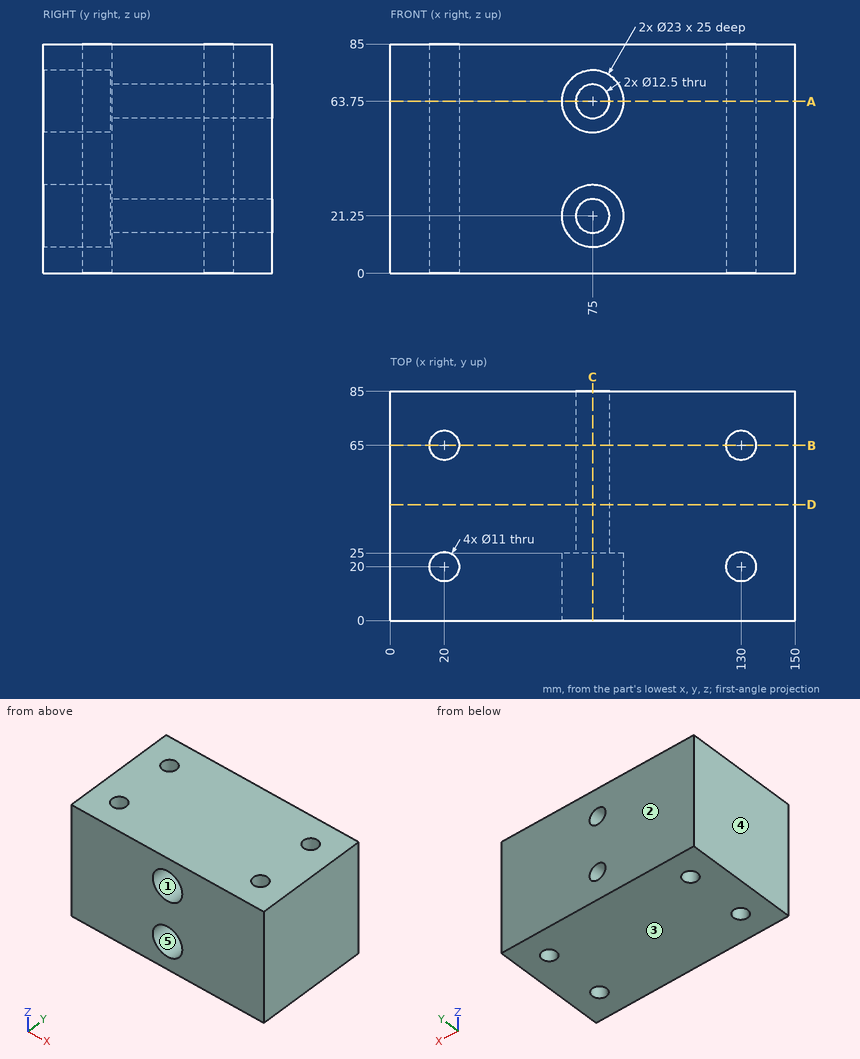
The figure shows three views and two pictorial views of one solid part (mm, origin at its lowest corner). Answer the questions. A direction names the side the tool comes from. Give positions to 0.01 mm unless a question says otherwise; leave off trailing zeros. Loops run counter-clockwise (first coordinate to the right, second up) from the corner with the lowest first, then second, coordinate; pieces in that order, holes last. Notation, with made-up numbers: (67.5, 88.25) -> (110.5, 88.25) arc R21 ccw to (110.5, 97.25) -> close; hole circle Ø9 at (-11.5, -13). An arc over 180 degrees is marked (long way). Use a Markdown table: item, result. Add a question column.
1. Flat-ended cylindrical pins translate along their axes: pin 1 Ø14.5 at (x, y) = (130, 65) entering from +Z; pin 2 Ø7 at (x, z) = (75.5, 25) entering from -Y. Find the tip coordinate at first contact, or state that the pin passes through.
2. For the marked faces 1 and 2, determine the directions among +Z, -Z, +X, -X, +Y, -Y from which every point of the face is accessible in a straight line to the end or side of a thin tool.
3. Section C-C on x = 75 is taken. Determine the outline of the cut face in (y, z), and give its area (4 significant figures).
4. Section A-A on z = 63.75 is taken. Determine the outline of the cut face in (x, y), and give its area (3 significant figures).
5. Section D-D on y = 43 is taken. Determine the outline of the cut face in (x, z).
6. Determine the mould class of the marked faces 3, 4 and 5 for opening direction Z: released by +Z, released by -Z, zero draft, split by the parting line, or undercut.
7. Section B-B on y = 65 is taken. Determine the outline of the cut face in (x, z), and give its area (3 significant figures).
8. Find the intervals of material crossed by probe 1 along X at (y, z) = (65.5, 47); probe 2 along Z at (x, y) = (75, 10.5); probe 3 along X at (y, z) = (63.5, 56), in increasing order.
Results below:
| question | item | result |
|---|---|---|
| 1 | pin 1 | stops at z = 85 |
| 1 | pin 2 | stops at y = 25 |
| 2 | face 1 | -Y |
| 2 | face 2 | +Z, -Z, +X, -X, +Y |
| 3 | outline | (0, 0) -> (85, 0) -> (85, 15) -> (25, 15) -> (25, 9.75) -> (0, 9.75) -> close; (0, 32.75) -> (25, 32.75) -> (25, 27.5) -> (85, 27.5) -> (85, 57.5) -> (25, 57.5) -> (25, 52.25) -> (0, 52.25) -> close; (0, 75.25) -> (25, 75.25) -> (25, 70) -> (85, 70) -> (85, 85) -> (0, 85) -> close |
| 3 | area | 4,575 mm^2 |
| 4 | outline | (0, 0) -> (63.5, 0) -> (63.5, 25) -> (68.75, 25) -> (68.75, 85) -> (0, 85) -> close; (81.25, 25) -> (86.5, 25) -> (86.5, 0) -> (150, 0) -> (150, 85) -> (81.25, 85) -> close; hole circle Ø11 at (20, 20); hole circle Ø11 at (20, 65); hole circle Ø11 at (130, 20); hole circle Ø11 at (130, 65) |
| 4 | area | 11,000 mm^2 |
| 5 | outline | (0, 0) -> (150, 0) -> (150, 85) -> (0, 85) -> close; hole circle Ø12.5 at (75, 21.25); hole circle Ø12.5 at (75, 63.75) |
| 6 | face 3 | released by -Z |
| 6 | face 4 | zero draft |
| 6 | face 5 | undercut |
| 7 | outline | (0, 0) -> (14.5, 0) -> (14.5, 85) -> (0, 85) -> close; (25.5, 0) -> (124.5, 0) -> (124.5, 85) -> (25.5, 85) -> close; (135.5, 0) -> (150, 0) -> (150, 85) -> (135.5, 85) -> close; hole circle Ø12.5 at (75, 21.25); hole circle Ø12.5 at (75, 63.75) |
| 7 | area | 10,600 mm^2 |
| 8 | probe 1 | x = 0 to 14.52, 25.48 to 124.52, 135.48 to 150 |
| 8 | probe 2 | z = 0 to 9.75, 32.75 to 52.25, 75.25 to 85 |
| 8 | probe 3 | x = 0 to 14.71, 25.29 to 124.71, 135.29 to 150 |
